from build123d import *

# Parameters (mm, degrees)
CUT_SKETCH_R     = 7.62
CENTER_CUT_DEPTH = 62.401577748
FILLET_2_R       = 3.175


with BuildPart() as part:
    # Revolve Sketch → Revolve 2 (revolve)
    with BuildSketch(Plane(origin=(0, 0, 0), x_dir=(0, 0, -1), z_dir=(1, 0, 0))):
        Polygon((0, 0), (0, 41.275), (-3.175, 41.275), (-3.175, 12.7), (-19.05, 12.7), (-19.05, 0), align=None)
    revolve(axis=Axis((0, 0, 0), (0, 0, 1)))

    # Cut Sketch → Center Cut (cut, through all)
    with BuildSketch(Plane.XY.offset(19.05)):
        Circle(CUT_SKETCH_R)
    extrude(amount=-CENTER_CUT_DEPTH, mode=Mode.SUBTRACT)

    # Fillet 2
    fillet_2_edges = [part.edges().sort_by_distance(p)[0] for p in [
        (0, -12.7, 3.175),
    ]]
    fillet(fillet_2_edges, radius=FILLET_2_R)


solid = part.part
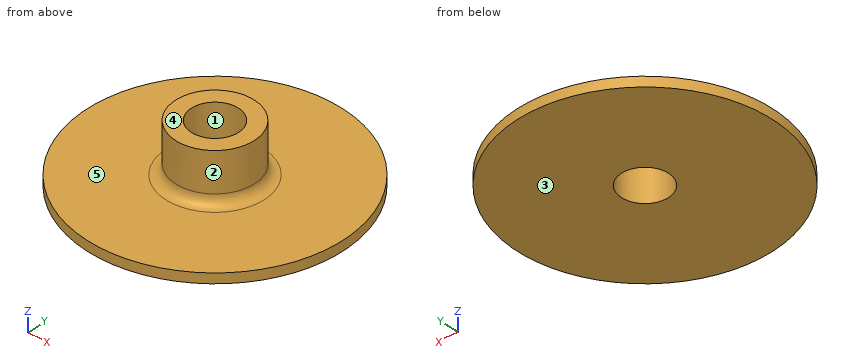
Verification items for the finished model (mm, model axes). Face numbers are marked on the shaded views. A direction names the side the tool comes from. Round coordinates to 2 decimals unless told otherwise and drop trailing zeros. Loops run counter-clockwise (first coordinate to the right, second up) from the corner with the lowest first, then second, coordinate; pieces in that order, holes last. Notation, with made-up numbers: (-38.75, -6) - (12.25, -6) arc R15 cw to (12.25, 16) - close; hole circle Ø4 at (87.25, 77.5). An arc over 180 degrees is marked (long way). Write item = value, one per line.
Q1. Tool access check on the marked faces 4 and 5. Record the directions out of +Z, -Z, +X, -X, +Y, -Y that give a thin tool (end or side, any length) a straight path to the whole face; none if there is none.
Here are the results:
face_4 = +Z, +X, -X, +Y, -Y
face_5 = +Z
Q2. Mould release check, pull along Y, two halves, no side actions. Record for the marked faces 1, 2 and 3: +Y half, -Y half, draft (parallel to the pull), parting line (faces both ways), or undercut.
Here are the results:
face_1 = undercut
face_2 = parting line
face_3 = draft
Q3. Material ranges on L1, parallel to Y at x = 0, z = 10; L2, parallel to Z at x = 26.5, y = -30.5 (3 decimals); L3, parallel to Y at x = 7, z = 6.25, recorded low to high.
Here are the results:
L1 = -12.7 to -7.62, 7.62 to 12.7
L2 = 0 to 3.175
L3 = -10.6 to -3.01, 3.01 to 10.6
Q4. Sectioned sample at D-D on y = 17.5. Record the boundary of the cut face in (x, z) (3 decimals), plus the area to 3 significant figures.
Here are the results:
outline = (-37.381, 0) - (37.381, 0) - (37.381, 3.175) - (-37.381, 3.175) - close
area = 237 mm^2
Q5. Depth check by flat-ended pin: pin 1 (3 mm diameter, centred on x = -1, y = 14.5, fed in from +Z); pin 2 (2 mm diameter, centred on x = 6, y = -22, fed in from +Z) (3 decimals); pin 3 (1 mm diameter, centred on x = 5, z = 2, fed in from -Y). Enter the tip coordinate at first touch or a pass-through.
Here are the results:
pin_1 = 4.93
pin_2 = 3.175
pin_3 = -41.03
Q6. Sectioned sample at A-A on x = 0. Record the boundary of the cut face in (y, z) (3 decimals), plus the area to 3 significant figures.
Here are the results:
outline = (-41.275, 0) - (-7.62, 0) - (-7.62, 19.05) - (-12.7, 19.05) - (-12.7, 6.35) arc R3.175 cw to (-15.875, 3.175) - (-41.275, 3.175) - close; (7.62, 0) - (41.275, 0) - (41.275, 3.175) - (15.875, 3.175) arc R3.175 cw to (12.7, 6.35) - (12.7, 19.05) - (7.62, 19.05) - close
area = 379 mm^2
Q7. Sectioned sample at C-C on z = 9.25. Record the boundary of the cut face in (x, y).
Here are the results:
outline = circle Ø25.4 at (0, 0); hole circle Ø15.24 at (0, 0)
